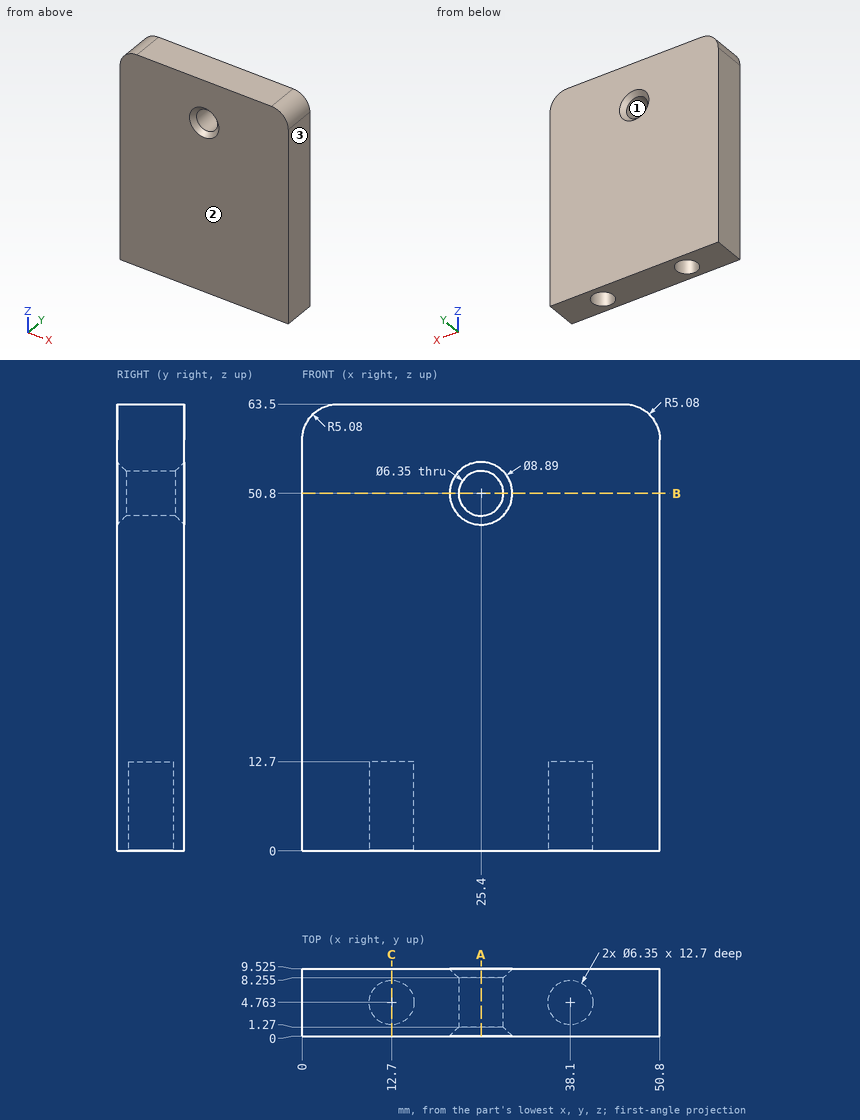
Job drawing, mm, ordinate dimensions from the low corner. One solid piece. Coordinates: 2 decimals unless noted, no trailing zeros. Order: outer loops, then holes, each group sorted by start corner. A loop starts at its lowest first (then second) coordinate and runs counter-clockwise, first axis right, second up. Notation, with made-up numbers: (66.5, 65.25) -> (80.5, 65.25) arc R18 ccw to (80.5, 100.25) -> close; hole circle Ø8 at (52.25, -37.75). An arc over 180 degrees is marked (long way). Return JSON: item names as keys, results as strings. Group by question number.
Item 1: Saw through at A-A on x = 25.4. Write the cut outline in (y, z) (1 decimal), then the cut area to 3 significant figures.
Item 2: Wall check: line 1 along Y through (x, z) = (38, 7) (1 decimal); line 2 along X through (y, z) = (3.25, 51); line 3 along Z through (x, y) = (25, 1.25). Give the ranges that are in metal, low to high. Write a range as [from, to].
Item 3: Saw through at B-B on z = 50.8. Write the cut outline in (x, y) (1 decimal).
Item 4: Pull direction X, two halves, no side cores. Call the marked faces 1, 2 and 3: pulls with the +X half, pulls with the -X half, needs draft (parallel to the pull), parting line crosses it, or undercut.
Item 5: Saw through at C-C on x = 12.7. Write the cut outline in (y, z) (1 decimal), then the cut area to 3 significant figures.
Item 6: Flat gauge pin, fed straight in: P1, Ø4, axis at x = 12.7, y = 4.76, coming from the -Z side. Where does the tip first touch, or does it go through?
Values found:
{
 "1": {"outline": "(0, 0) -> (9.5, 0) -> (9.5, 46.4) -> (8.3, 47.6) -> (1.3, 47.6) -> (0, 46.4) -> close; (0, 55.2) -> (1.3, 54) -> (8.3, 54) -> (9.5, 55.2) -> (9.5, 63.5) -> (0, 63.5) -> close", "area": "541 mm2"},
 "2": {"line 1": "y = [0, 1.6], [7.9, 9.5]", "line 2": "x = [0, 22.23], [28.57, 50.8]", "line 3": "z = [0, 47.63], [53.97, 63.5]"},
 "3": {"outline": "(0, 0) -> (21, 0) -> (22.2, 1.3) -> (22.2, 8.3) -> (21, 9.5) -> (0, 9.5) -> close; (28.6, 1.3) -> (29.8, 0) -> (50.8, 0) -> (50.8, 9.5) -> (29.8, 9.5) -> (28.6, 8.3) -> close"},
 "4": {"face 1": "undercut", "face 2": "needs draft", "face 3": "pulls with the +X half"},
 "5": {"outline": "(0, 0) -> (1.6, 0) -> (1.6, 12.7) -> (7.9, 12.7) -> (7.9, 0) -> (9.5, 0) -> (9.5, 63.5) -> (0, 63.5) -> close", "area": "524 mm2"},
 "6": {"P1": "stops at z = 12.7"}
}
